```python
from build123d import *

# Parameters (mm, degrees)
SKETCH2_R          = 1.237013061
CUT_EXTRUDE1_DEPTH = 36.580893749
CIRPATTERN1_COUNT  = 3
FILLET2_R          = 3
FILLET3_R          = 1


with BuildPart() as part:
    # Sketch1 → Revolve1 (revolve)
    with BuildSketch(Plane(origin=(0, 0, 0), x_dir=(0, 0, -1), z_dir=(1, 0, 0))):
        Polygon((0, 0), (0, -5), (-11, -5), (-11, -7), (3.8, -7), (5.8, -5), (5.8, 0), align=None)
    revolve(axis=Axis((0, 1.658614865, -9), (0, -1, 0)))

    # Sketch2 → Cut-Extrude1 (cut, through all)
    with BuildSketch(Plane(origin=(0, -5, 0), x_dir=(1, 0, 0), z_dir=(0, 1, 0))):
        with Locations(Location((0, 23.5, 0), (0, 0, 270))):
            Circle(SKETCH2_R)
    cut_extrude1 = extrude(amount=-CUT_EXTRUDE1_DEPTH, mode=Mode.SUBTRACT)

    # CirPattern1: Cut-Extrude1 ×3 about axis
    cirpattern1_axis = Axis((0, 0, -9), (0, 1, 0))
    for i in range(1, CIRPATTERN1_COUNT):
        add(cut_extrude1.rotate(cirpattern1_axis, i * 360 / CIRPATTERN1_COUNT), mode=Mode.SUBTRACT)

    # Fillet2
    fillet2_edges = [part.edges().sort_by_distance(p)[0] for p in [
        (0, -5, -18),
    ]]
    fillet(fillet2_edges, radius=FILLET2_R)

    # Fillet3
    fillet3_edges = [part.edges().sort_by_distance(p)[0] for p in [
        (0, -5, -12.2),
    ]]
    fillet(fillet3_edges, radius=FILLET3_R)


solid = part.part
```
Check sheet for the modelled part. Datum: model origin and axes. Units: mm. A direction names the side the tool comes from. Coordinates: 2 decimals unless noted, no trailing zeros. Write each loop counter-clockwise with the first axis right and the second up, starting at its lowest first coordinate (ties: lowest second). Pieces come first, ordered by that corner, then holes. Notation, with made-up numbers: M 14.25,-22.75 L 71.25,-22.75 A29 ccw 71.25,-2.75 Z; hole C -1,-19 d11. An arc over 180 degrees is marked long. Use one line per item in the form item = value.
Item 1: Sectioned sample at A-A, the plane z = -23.5. Record the cut outline in (x, y).
Answer below:
outline = M -13.77,-7 L -1.24,-7 L -1.24,-5 L -13.77,-5 Z; M 1.24,-7 L 13.77,-7 L 13.77,-5 L 1.24,-5 Z
Item 2: Sectioned sample at B-B, the plane y = -0.75. Record the cut outline in (x, z).
Answer below:
outline = C 0,-9 d18; hole C 0,-9 d6.4
Item 3: Release check for a two-part mould opening along Z. For faces 1 (the face through (4, -7, -5)), 2 (the face through (13.784, -5.986, -1.911)), 3 (the face through (-8.923, -1.014, -10.172)) record: pulls with the +Z half, pulls with the -Z half, needs draft (parallel to the pull), parting line crosses it, or undercut.
Answer below:
face_1 = needs draft
face_2 = undercut
face_3 = parting line crosses it
Item 4: Sectioned sample at D-D, the plane x = 17.5. Record the cut outline in (y, z), and give its area (3 significant figures).
Answer below:
outline = M -7,-18.68 L -5,-18.68 L -5,0.68 L -7,0.68 Z
area = 38.7 mm^2
Item 5: Material ranges on L1, parallel to X at y = -5.7, z = -1.75; L2, parallel to Y at x = 10, z = -18; L3, parallel to X at y = -5.75, z = -23.5, recorded low to high. Write a range as from..to.
Answer below:
L1 = -18.64..-13.79, -11.32..11.32, 13.79..18.64
L2 = -7..-5
L3 = -13.77..-1.24, 1.24..13.77
Item 6: Set-up check for faces 4 (the face through (9, -5, -18)), 5 (the face through (19.524, -6.014, -13.336)): record each of +Z, -Z, +X, -X, +Y, -Y from which the full face is reachable in a straight line by a thin tool's end or side.
Answer below:
face_4 = +Y
face_5 = +Y, -Y
Item 7: Sectioned sample at C-C, the plane y = -6.5. Record the cut outline in (x, z).
Answer below:
outline = C 0,-9 d40; hole C -12.56,-1.75 d2.47; hole C 0,-9 d9.4; hole C 0,-23.5 d2.47; hole C 12.56,-1.75 d2.47
Item 8: Gauge pin test, flat ends, axial feed: pin 1 Ø4 at (x, y) = (-1.5, -4) entering from -Z; pin 2 Ø2 at (x, y) = (1.5, -3.5) entering from +Z; pin 3 Ø4 at (y, z) = (-1, -16) entering from +X. Record the tip position at first contact, or that the pin passes through.
Answer below:
pin_1 = -29
pin_2 = 1.24
pin_3 = 7.48
